Verification items for this drawing (mm, ordinates from the low corner). A direction names the side the tool comes from. Give positions to 0.01 mm unless a question says otherwise; leave off trailing zeros. Loops run counter-clockwise (first coordinate to the right, second up) from the corner with the lowest first, then second, coordinate; pieces in that order, holes last. Notation, with made-up numbers: (70.25, 2.5) -> (108.25, 2.5) arc R25 cw to (108.25, 34.5) -> close; hole circle Ø1 at (68, 55.5). An arc over 180 degrees is marked (long way). Answer as a JSON object with one key per item and string values.
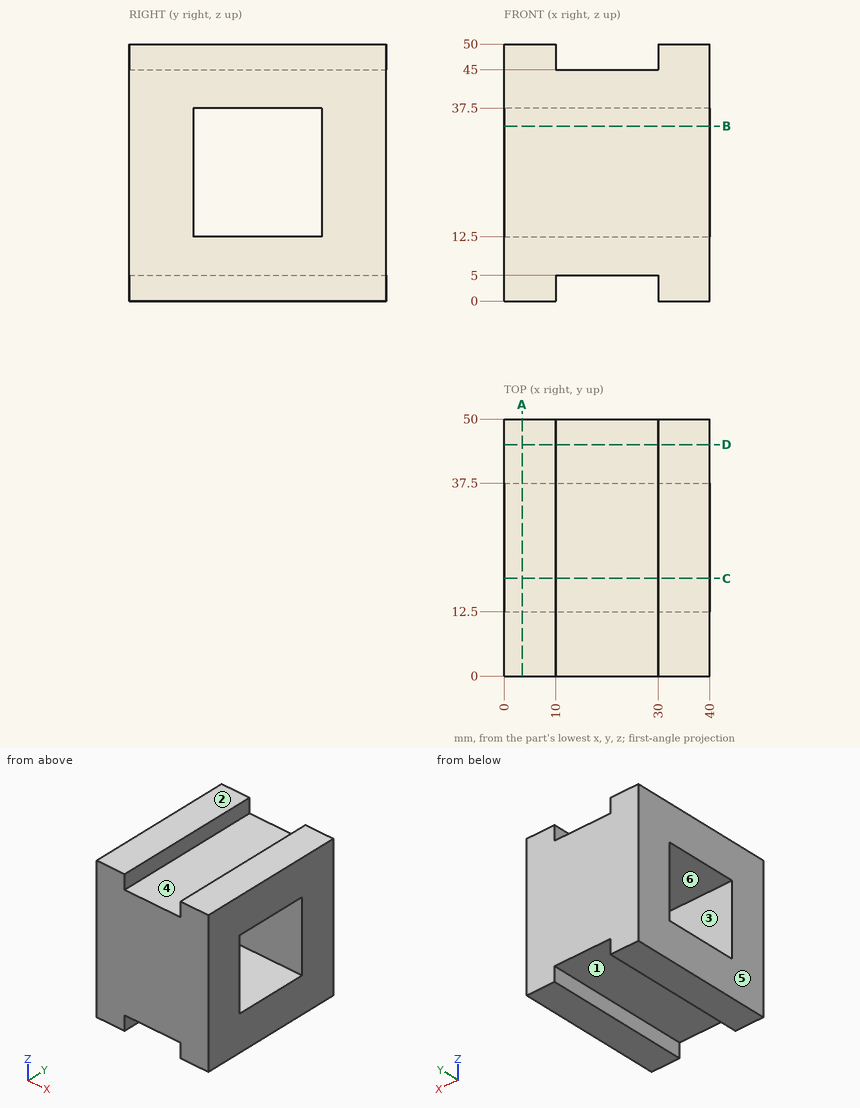
1) Tool access check on the marked faces 1, 2 and 3. Record the directions out of +Z, -Z, +X, -X, +Y, -Y that give a thin tool (end or side, any length) a straight path to the whole face; none if there is none.
Geometry check:
{"face 1": "-Z, +Y, -Y", "face 2": "+Z, +X, -X, +Y, -Y", "face 3": "+X, -X"}
2) Section check D-D on y = 45. Record the cut outline in (x, z).
Geometry check:
{"outline": "(0, 0) -> (10, 0) -> (10, 5) -> (30, 5) -> (30, 0) -> (40, 0) -> (40, 50) -> (30, 50) -> (30, 45) -> (10, 45) -> (10, 50) -> (0, 50) -> close"}
3) Section check C-C on y = 19. Record the cut outline in (x, z), plus the area to 3 significant figures.
Geometry check:
{"outline": "(0, 0) -> (10, 0) -> (10, 5) -> (30, 5) -> (30, 0) -> (40, 0) -> (40, 12.5) -> (0, 12.5) -> close; (0, 37.5) -> (40, 37.5) -> (40, 50) -> (30, 50) -> (30, 45) -> (10, 45) -> (10, 50) -> (0, 50) -> close", "area": "800 mm2"}
4) Section check A-A on x = 3.5. Record the cut outline in (y, z).
Geometry check:
{"outline": "(0, 0) -> (50, 0) -> (50, 50) -> (0, 50) -> close; hole (12.5, 12.5) -> (37.5, 12.5) -> (37.5, 37.5) -> (12.5, 37.5) -> close"}
5) Draft check along X on the marked faces 4, 5 and 6. Enter one of: pulls with the +X half, pulls with the -X half, needs draft (parallel to the pull), parting line crosses it, or undercut.
Geometry check:
{"face 4": "undercut", "face 5": "pulls with the -X half", "face 6": "needs draft"}
6) Depth check by flat-ended pin: P1, Ø10, axis at x = 21.5, y = 25.5, coming from the -Z side; P2, Ø10, axis at x = 19.5, y = 15, coming from the +Z side. Enter the tip coordinate at first touch or a pass-through.
Geometry check:
{"P1": "stops at z = 5", "P2": "stops at z = 45"}
7) Section check B-B on z = 34. Record the cut outline in (x, y), plus the area to 3 significant figures.
Geometry check:
{"outline": "(0, 0) -> (40, 0) -> (40, 12.5) -> (0, 12.5) -> close; (0, 37.5) -> (40, 37.5) -> (40, 50) -> (0, 50) -> close", "area": "1,000 mm2"}
8) Material ranges on line 1 along Z through (x, y) = (7.5, 21); line 2 along Z through (x, y) = (27.5, 36.5), recorded low to high. Write a range as from..to.
Geometry check:
{"line 1": "z = 0..12.5, 37.5..50", "line 2": "z = 5..12.5, 37.5..45"}
